Read the model definition and answer for the solid it produces. Units are mm, in the model's axes. Face numbers are marked on the shaded views. A direction names the side the tool comes from. Give positions to 0.01 mm unless a question says otherwise; leave off trailing zeros. Write each loop counter-clockwise with the first axis right and the second up, starting at its lowest first coordinate (ties: lowest second). Pieces come first, ordered by that corner, then holes. Notation, with made-up numbers: (51.25, -30) -> (92.25, -30) arc R16 ccw to (92.25, -2) -> close; hole circle Ø4 at (12.5, 56). An arc over 180 degrees is marked (long way). Use a Markdown table: item, result.
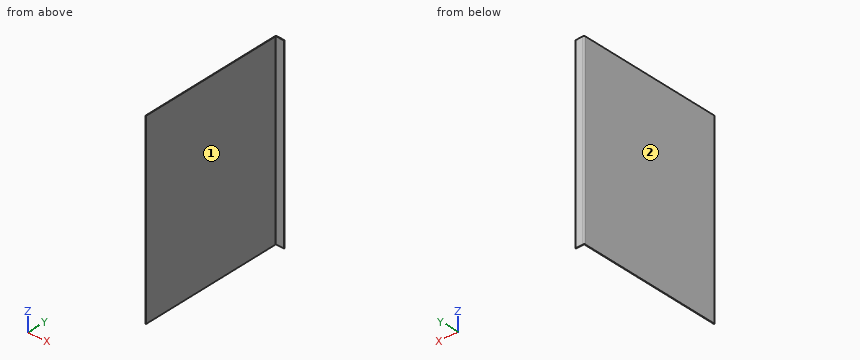
Autodesk Inventor part; units mm, degrees
ref_plane "YZ Plane" through (0, 0, 0) normal (1, 0, 0) x (0, 1, 0)
ref_plane "XZ Plane" through (0, 0, 0) normal (0, 1, 0) x (-1, 0, 0)
ref_plane "XY Plane" through (0, 0, 0) normal (0, 0, 1) x (1, 0, 0)
sketch "Sketch29" plane through (0, 0, 0) normal (1, 0, 0) x (0, 1, 0)
  line L0 (0, 0) -> (1657.35, 0)
  line L1 (1657.35, 0) -> (1657.35, 2107.692)
  line L2 (1657.35, 2107.692) -> (0, 2107.692)
  line L3 (0, 2107.692) -> (0, 0)
  dimension "d230" = 2107.692
  dimension "d231" = 1657.35
extrude "Plate26" add sketch "Sketch29" along normal blind 6.35
sketch "Sketch30" plane through (-0.2216, 1651.0039, 2107.692) normal (0.0348995, 0.9993908, 0) x (-0.9993908, 0.0348995, 0)
  line L0 (0, -2107.692) -> (0, 0)
  line L1 (0, 0) -> (-101.6, 0)
  line L2 (-101.6, 0) -> (-101.6, -2107.692)
  line L3 (-101.6, -2107.692) -> (0, -2107.692)
edge flange "Flange23" height 101.6 angle 92 thickness 6.35 bend radius 6.35 thickness toward (0.0348995, 0.9993908, 0) relief tear relief width 6.35 relief depth 3.175 edges at (6.35, 1657.35, 1053.846) wall of the first edge with corners at (-0.2216, 1651.0039, 0) (-0.2216, 1651.0039, 2107.692) (101.3165, 1647.4581, 2107.692) (101.3165, 1647.4581, 0)
bend "Bend23"
corner "Corner22"
equation "\"d230\" = LARGO"
equation "\"d231\" = ALTO"
equation "\"d237\" = LARGOF"
equation "\"d238\" = ANGULOF"
equation "\"BendRadius\" = Thickness"
equation "\"BendReliefWidth\" = Thickness"
equation "\"BendReliefDepth\" = 0.5 * Thickness"
equation "\"CornerReliefSize\" = 4 * Thickness"
equation "\"MinimumRemnant\" = 2 * Thickness"
equation "\"TransitionRadius\" = BendRadius"
equation "\"JacobiRadiusSize\" = BendRadius"
equation "\"GapSize\" = Thickness"
equation "\"LARGO\" = 2107.692"
equation "\"ALTO\" = 1657.35"
equation "\"LARGOF\" = 101.6"
equation "\"ANGULOF\" = 92deg"
properties part number "BackWallTop" material "Carbon Steel - A36"
Item 1: Straight lines are drawn through the part: line 1 along X through (y, z) = (1368.5, 681); line 2 along Y through (x, z) = (18, 1683.5); line 3 along Y through (x, z) = (16, 1387). For each, find the intervals that lie inside material, in ascending order. Write a range as [from, to].
Return value:
| item | result |
|---|---|
| line 1 | [0, 6.35] |
| line 2 | [1650.37, 1656.72] |
| line 3 | [1650.44, 1656.79] |
Item 2: A cutting plane is placed at A-A (z = 1074.5). Give the vertices of the cut face in (x, y), then the cut area to 3 significant figures.
Return value:
| item | result |
|---|---|
| outline | (0, 0) -> (6.35, 0) -> (6.35, 1644.2) arc R6.35 cw to (12.92, 1650.54) -> (101.32, 1647.46) -> (101.54, 1653.8) -> (13.14, 1656.89) arc R12.7 ccw to (0, 1644.2) -> close |
| area | 11,100 mm^2 |
Item 3: A tool of negligible diameter and unlimited length cuts with its end or side. For the marked faces 1 and 2, from which of +Z, -Z, +X, -X, +Y, -Y can it reach the whole face along a straight path? Write none if from no direction.
Return value:
| item | result |
|---|---|
| face 1 | +Z, -Z, +X, -Y |
| face 2 | +Z, -Z, -X, +Y, -Y |
Item 4: A cutting plane is placed at C-C (x = 44.5). Give the vertices of the cut face in (y, z), then the cut area to 3 significant figures.
Return value:
| item | result |
|---|---|
| outline | (1649.44, 0) -> (1655.8, 0) -> (1655.8, 2107.69) -> (1649.44, 2107.69) -> close |
| area | 13,400 mm^2 |
Item 5: A cutting plane is placed at B-B (y = 161). Give the vertices of the cut face in (x, z).
Return value:
| item | result |
|---|---|
| outline | (0, 0) -> (6.35, 0) -> (6.35, 2107.69) -> (0, 2107.69) -> close |
Item 6: Each of these flat-tipped pins is pushed along its axis until it touches: P1, Ø8, axis at x = 76, z = 323, coming from the +Y side; P2, Ø8, axis at x = 77, z = 1740.5, coming from the -Y side; P3, Ø6, axis at x = 54, z = 1592.5, coming from the -Y side. Where does it stop, or does it pass through?
Return value:
| item | result |
|---|---|
| P1 | y = 1654.84 |
| P2 | y = 1648.17 |
| P3 | y = 1649.01 |
